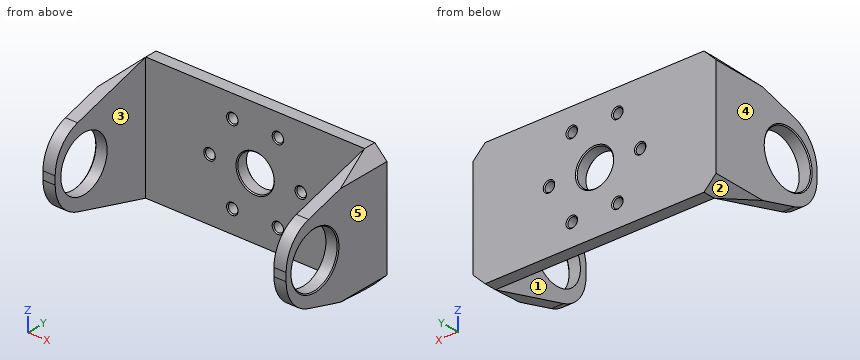
```python
from build123d import *

# Parameters (mm, degrees)
SKETCH1_W                      = 114.3
SKETCH1_H                      = 64.77
BOSS_EXTRUDE1_DEPTH            = 6.35
BOSS_EXTRUDE2_DEPTH            = 6.35
BOSS_EXTRUDE3_DEPTH            = 6.35
HOLE1_D                        = 18.9738
HOLE1_DEPTH                    = 6.35
F_9_0_196_DIAMETER_HOLE1_D     = 4.9784
F_9_0_196_DIAMETER_HOLE1_DEPTH = 62.23
F_9_0_196_DIAMETER_HOLE2_D     = 4.9784
F_9_0_196_DIAMETER_HOLE2_DEPTH = 6.35
HOLE2_D                        = 28.575
HOLE2_DEPTH                    = 6.35
HOLE3_D                        = 28.575
HOLE3_DEPTH                    = 127
CHAMFER1_SIZE                  = 6.35
CHAMFER2_SIZE                  = 0.508
FILLET1_R                      = 19.05


with BuildPart() as part:
    # Sketch1 → Boss-Extrude1 (new body)
    with BuildSketch(Plane(origin=(0, 6.35, 0), x_dir=(1, 0, 0), z_dir=(0, 1, 0))):
        Rectangle(SKETCH1_W, SKETCH1_H)
    extrude(amount=-BOSS_EXTRUDE1_DEPTH)

    # Sketch2 → Boss-Extrude2 (add)
    with BuildSketch(Plane(origin=(57.15, 0, 0), x_dir=(0, 0, -1), z_dir=(1, 0, 0))):
        Polygon((-32.385, 6.35), (32.385, 6.35), (32.385, 0), (16.51, -55.88), (-16.51, -55.88), (-32.385, 0), align=None)
    extrude(amount=BOSS_EXTRUDE2_DEPTH)

    # Sketch3 → Boss-Extrude3 (add)
    with BuildSketch(Plane.ZY.offset(57.15)):
        Polygon((32.385, 0), (16.51, -55.88), (-16.51, -55.88), (-32.385, 0), (-32.385, 6.35), (32.385, 6.35), align=None)
    extrude(amount=BOSS_EXTRUDE3_DEPTH)

    # Hole1
    with Locations(Plane(origin=(0, 0, 0), x_dir=(-1, 0, 0), z_dir=(0, -1, 0))):
        with Locations((0, 0)):
            Hole(HOLE1_D / 2, depth=HOLE1_DEPTH)

    # #9 (0.196) Diameter Hole1
    with Locations(Plane(origin=(0, 6.35, 0), x_dir=(1, 0, 0), z_dir=(0, 1, 0))):
        with Locations((11.90625, 20.622229928)):
            Hole(F_9_0_196_DIAMETER_HOLE1_D / 2, depth=F_9_0_196_DIAMETER_HOLE1_DEPTH)

    # #9 (0.196) Diameter Hole2
    with Locations(Plane(origin=(0, 0, 0), x_dir=(-1, 0, 0), z_dir=(0, -1, 0))):
        with Locations((-23.8125, 0), (-11.90625, -20.622229928), (11.90625, -20.622229928), (23.8125, 0), (11.90625, 20.622229928)):
            Hole(F_9_0_196_DIAMETER_HOLE2_D / 2, depth=F_9_0_196_DIAMETER_HOLE2_DEPTH)

    # Hole2
    with Locations(Plane.ZY.offset(63.5)):
        with Locations((0, -38.1)):
            Hole(HOLE2_D / 2, depth=HOLE2_DEPTH)

    # Hole3
    with Locations(Plane(origin=(63.5, 0, 0), x_dir=(0, 0, -1), z_dir=(1, 0, 0))):
        with Locations((0, -38.1)):
            Hole(HOLE3_D / 2, depth=HOLE3_DEPTH)

    # Chamfer1
    chamfer1_edges = [part.edges().sort_by_distance(p)[0] for p in [
        (63.5, 3.175, -32.385),
        (63.5, 3.175, 32.385),
        (-63.5, 3.175, -32.385),
        (-63.5, 3.175, 32.385),
    ]]
    chamfer(chamfer1_edges, length=CHAMFER1_SIZE)

    # Chamfer2
    chamfer2_edges = [part.edges().sort_by_distance(p)[0] for p in [
        (-9.4869, 0, 0),
        (-9.4869, 6.35, 0),
        (14.39545, 0, -20.622229928),
        (14.39545, 6.35, -20.622229928),
        (-14.39545, 0, -20.622229928),
        (-14.39545, 6.35, -20.622229928),
        (-26.3017, 0, 0),
        (-26.3017, 6.35, 0),
        (-14.39545, 0, 20.622229928),
        (-14.39545, 6.35, 20.622229928),
        (9.41705, 0, 20.622229928),
        (9.41705, 6.35, 20.622229928),
        (21.3233, 0, 0),
        (21.3233, 6.35, 0),
        (-63.5, -38.1, 14.2875),
        (63.5, -38.1, -14.2875),
    ]]
    chamfer(chamfer2_edges, length=CHAMFER2_SIZE)

    # Fillet1
    fillet1_edges = [part.edges().sort_by_distance(p)[0] for p in [
        (60.325, -55.88, 16.51),
        (60.325, -55.88, -16.51),
        (-60.325, -55.88, -16.51),
        (-60.325, -55.88, 16.51),
    ]]
    fillet(fillet1_edges, radius=FILLET1_R)


solid = part.part
```
CAD build for the part. Positions are in the model's coordinates, mm. Face numbers are marked on the shaded views. A direction names the side the tool comes from. Coordinates: 2 decimals unless noted, no trailing zeros. Loops run counter-clockwise (first coordinate to the right, second up) from the corner with the lowest first, then second, coordinate; pieces in that order, holes last. Notation, with made-up numbers: (13.25, -28.75) - (48.25, -28.75) arc R34 cw to (48.25, 3.25) - close; hole circle Ø3 at (-33, 45). An arc over 180 degrees is marked (long way). Return JSON: item names as keys, results as strings.
1. Band-saw the part on D-D (x = 18.5). Give the cut face in (y, z) (3 decimals).
Result:
{"outline": "(0, -32.385) - (6.35, -32.385) - (6.35, 32.385) - (0, 32.385) - close"}
2. Probe L1, parallel to Z at x = -12, y = 3.5 (3 decimals); L2, parallel to Y at x = -59.45, z = 0; L3, parallel to X at y = -15, z = -12. List the from-to ranges inside material, lowest first. Write a range as from..to.
Result:
{"L1": "z = -32.385..-23.11, -18.135..18.135, 23.11..32.385", "L2": "y = -55.88..-52.39, -23.81..6.35", "L3": "x = -63.5..-57.15, 57.15..63.5"}
3. 3-axis set-ups, long thin cutter, end or side, ignore diameter. For the marked faces 1 and 2: which of +Z, -Z, +X, -X, +Y, -Y reach the whole face in a straight line?
Result:
{"face 1": "+Z, -Z, -Y", "face 2": "-Z, -X, +Y, -Y"}
4. Band-saw the part on A-A (x = 0). Give the cut face in (y, z) (3 decimals).
Result:
{"outline": "(0, -32.385) - (6.35, -32.385) - (6.35, -9.995) - (5.842, -9.487) - (0.508, -9.487) - (0, -9.995) - close; (0, 9.995) - (0.508, 9.487) - (5.842, 9.487) - (6.35, 9.995) - (6.35, 32.385) - (0, 32.385) - close"}
5. Drop flat-ended pins along their axis: pin 1 (12 mm diameter, centred on y = -39.5, z = 12, fed in from -X); pin 2 (4 mm diameter, centred on x = 23.81, z = 0, fed in from -Y); pin 3 (6 mm diameter, centred on x = -32, z = -8.5, fed in from -Y). Give the stop position or say it passes through.
Result:
{"pin 1": "stops at x = -63.5", "pin 2": "passes through", "pin 3": "stops at y = 0"}
6. Mould opens along X. For the marked faces 3, 4 and 5 say: released by +X, released by -X, zero draft, split by the parting line, or undercut.
Result:
{"face 3": "undercut", "face 4": "released by -X", "face 5": "released by +X"}
7. Band-saw the part on B-B (z = 0). State how many separate pieces and enclosed holes the cut face has, and give its area (3 significant figures).
Result:
{"separate pieces": "6", "enclosed holes": "0", "area": "967 mm2"}
